Input: dimensioned drawing with shaded views. Units: mm. Origin: part minimum x, y, z. A direction names the side the tool comes from. Round coordinates to 2 decimals unless told otherwise and drop trailing zeros. Order: outer loops, then holes, each group sorted by start corner. A loop starts at its lowest first (then second) coordinate and runs counter-clockwise, first axis right, second up. Notation, with made-up numbers: M 70,32 L 78,32 A26 ccw 78,61 Z; hole C -15.75,18 d10. An arc over 180 degrees is marked long. Use one line per item in the form item = value. Start each with the question number.
Q1. Contact query for flat-ended pins moving along their axis: pin 1 (3 mm diameter, centred on y = 6.35, z = 9.525, fed in from +X); pin 2 (2.5 mm diameter, centred on x = 12.5, z = 8.5, fed in from -Y) (3 decimals); pin 3 (1 mm diameter, centred on x = 10.5, z = 1.5, fed in from -Y); pin 4 (1.5 mm diameter, centred on x = 3.5, y = 3.5, fed in from +Z). Output: stop coordinate, or through.
Q2. Section A-A (y = 6.35). Return the cut outline in (x, z), plus the area to 3 significant figures.
Q3. Pull-direction query (Z, two-part tool) for the marked faces 1, 2 and 3; classes: pulls with the +Z half, pulls with the -Z half, needs draft (parallel to the pull), parting line crosses it, or undercut.
Q4. Section B-B (x = 6.5). Return the cut outline in (y, z) (3 decimals).
Q5. Section D-D (y = 3). Return the cut outline in (x, z).
Q6. Section C-C (y = 9.75). Return the cut outline in (x, z), plus the area to 3 significant figures.
Q7. Reachability of the marked faces 4 and 5 from +Z, -Z, +X, -X, +Y, -Y: full face, straight path, thin tool, end or side. Return the list, or none.
Q8. Material intervals for probe 1 along Y at (x, z) = (15, 7.5) (3 decimals); probe 2 along Y at (x, z) = (8, 10.25); probe 3 along Y at (x, z) = (17.25, 10), sorted ascending.
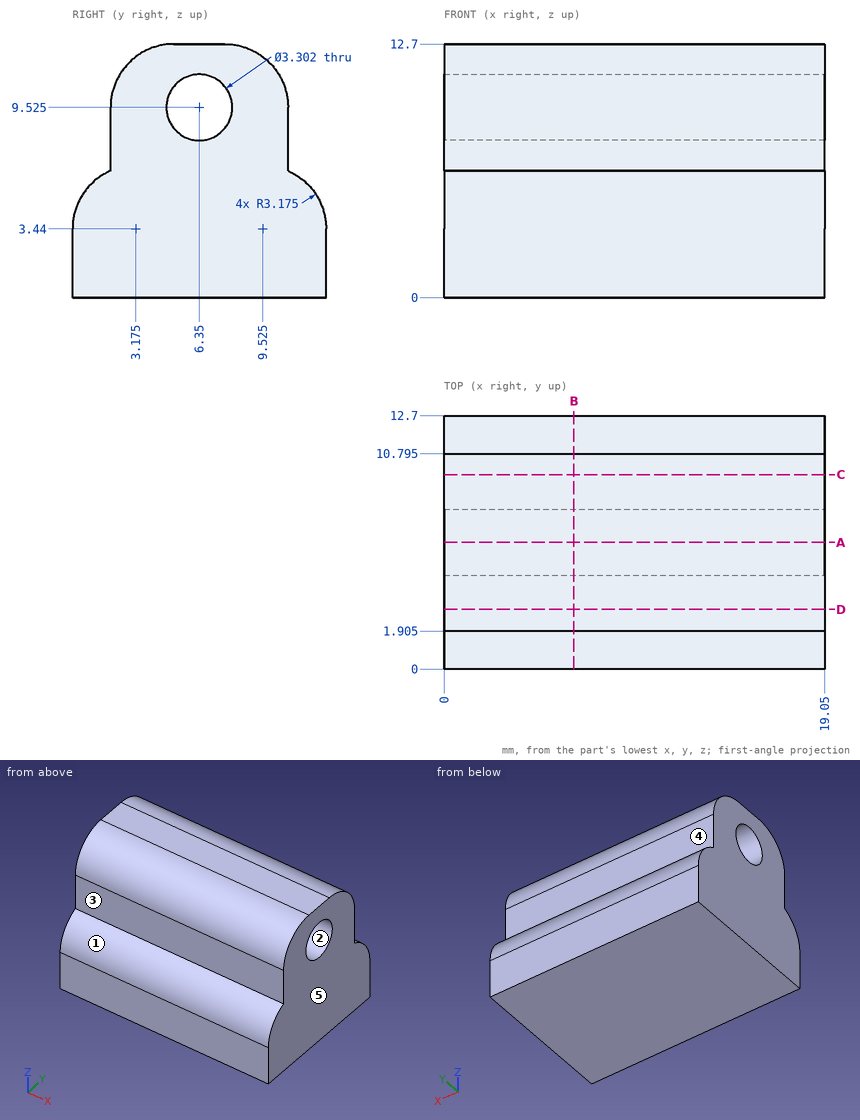
Results list:
q1.pin_1 = through
q1.pin_2 = 1.905
q1.pin_3 = 0
q1.pin_4 = 12.59
q2.outline = M 0,0 L 19.05,0 L 19.05,7.87 L 0,7.87 Z; M 0,11.18 L 19.05,11.18 L 19.05,12.7 L 0,12.7 Z
q2.area = 179 mm2
q3.face_1 = pulls with the +Z half
q3.face_2 = undercut
q3.face_3 = needs draft
q4.outline = M 0,0 L 12.7,0 L 12.7,3.44 A3.175 ccw 10.795,6.35 L 10.795,9.525 A3.175 ccw 7.62,12.7 L 5.08,12.7 A3.175 ccw 1.905,9.525 L 1.905,6.35 A3.175 ccw 0,3.44 Z; hole C 6.35,9.525 d3.302
q5.outline = M 0,0 L 19.05,0 L 19.05,11.92 L 0,11.92 Z
q6.outline = M 0,0 L 19.05,0 L 19.05,11.88 L 0,11.88 Z
q6.area = 226 mm2
q7.face_4 = +Z, +X, -X, +Y
q7.face_5 = +Z, -Z, +X, +Y, -Y
q8.probe_1 = 1.905 to 10.795
q8.probe_2 = 1.99 to 4.87, 7.83 to 10.71
q8.probe_3 = 1.94 to 4.77, 7.93 to 10.76
